The figure shows three views and two pictorial views of one solid part (mm, origin at its lowest corner). Answer the questions. A direction names the side the tool comes from. Coordinates: 2 decimals unless noted, no trailing zeros. Write each loop counter-clockwise with the first axis right and the second up, starting at its lowest first coordinate (ties: lowest second). Pieces come first, ordered by that corner, then holes. Notation, with made-up numbers: M 17,29 L 59,29 A8 cw 59,38 Z; hole C 46,62.5 d8. An arc over 180 degrees is marked long. Use CSV: the item, a comma, the result in double quotes.
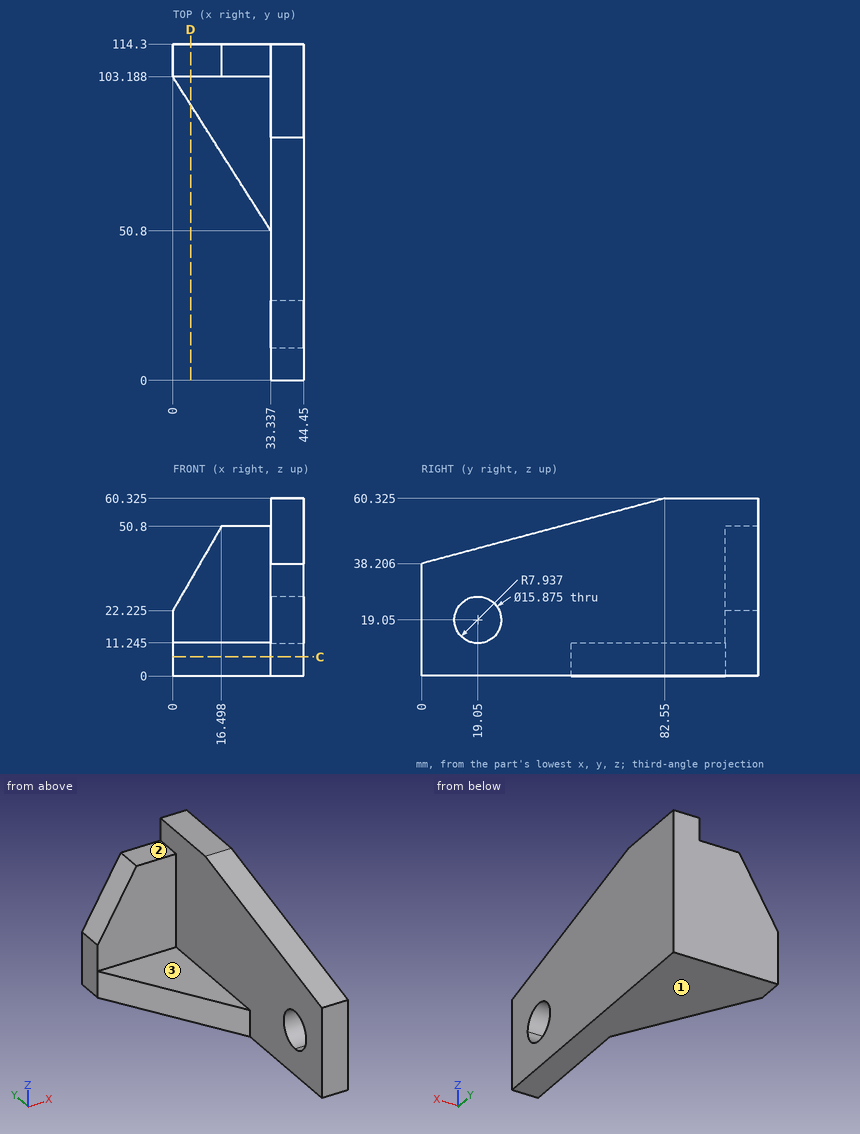
Item 1: Consider probe 1 along Y at (x, z) = (41, 19); probe 2 along X at (y, z) = (97, 24.5); probe 3 along Z at (x, y) = (38, 19.05). Determine where each line is inside the solid, lowest interval first.
Answer:
probe 1,"y = 0 to 11.11, 26.99 to 114.3"
probe 2,"x = 33.34 to 44.45"
probe 3,"z = 0 to 11.11, 26.99 to 43.31"
Item 2: Given pin 1 (16.5 mm diameter, centred on x = 10, y = 90, fed in from +Z) (1 decimal); pin 2 (1 mm diameter, centred on y = 45, z = 36.5, fed in from -X); pin 3 (10 mm diameter, centred on x = 23.5, z = 25.5, fed in from -Y), each flat-ended and moving along its own axis, determine where each tip first touches the part or whether it passes through.
Answer:
pin 1,"stops at z = 11.2"
pin 2,"stops at x = 33.34"
pin 3,"stops at y = 103.19"
Item 3: A tool of negligible diameter and unlimited length cuts with its end or side. For the marked faces 1, 2 and 3, from which of +Z, -Z, +X, -X, +Y, -Y can it reach the whole face along a straight path? Write none if from no direction.
Answer:
face 1,"-Z, +X, -X, +Y, -Y"
face 2,"+Z, -X, +Y, -Y"
face 3,"+Z, -X, -Y"
Item 4: The part is cut by section C-C (z = 6.5). Write down the section's boundary in (x, y), then the cut area to 3 significant figures.
Answer:
outline,"M 0,103.19 L 33.34,50.8 L 33.34,0 L 44.45,0 L 44.45,114.3 L 0,114.3 Z"
area,"2,510 mm2"
Item 5: The part is cut by section D-D (x = 6). Write down the section's boundary in (y, z) (1 decimal).
Answer:
outline,"M 93.8,0 L 114.3,0 L 114.3,32.6 L 103.2,32.6 L 103.2,11.2 L 93.8,11.2 Z"
